Could you check a few things on this model? Use its own coordinates, in mm. Face numbers are marked on the shaded views. Round coordinates to 2 decimals unless told otherwise and drop trailing zeros. Write each loop counter-clockwise with the first axis right and the second up, starting at its lowest first coordinate (ties: lowest second). Pieces come first, ordered by that corner, then holes. Notation, with made-up numbers: M 13,43.5 L 53,43.5 A20 cw 53,73.5 Z; hole C -25,18.5 d7. An arc over 180 degrees is marked long. One line per question, with ' | ' between items. Start each with the question number.
```python
from build123d import *

# Parameters (mm, degrees)
SKETCH1_W             = 76.2
SKETCH1_H             = 50.8
SKETCH1_R             = 1.397
BOSS_EXTRUDE1_DEPTH   = 8.89
FILLET1_R             = 5.08
SKETCH2_R             = 2.370137615
CUT_EXTRUDE1_DEPTH    = 47.645493887
SKETCH3_R             = 5.08
CUT_EXTRUDE2_DEPTH    = 5.08
SKETCH4_W             = 50.8
SKETCH4_H             = 3.81
CUT_EXTRUDE3_DEPTH    = 47.645493887
FILLET2_R             = 1.905
F_6_32_TAPPED_HOLE1_D = 2.7051


with BuildPart() as part:
    # Sketch1 → Boss-Extrude1 (new body)
    with BuildSketch(Plane.XY):
        Rectangle(SKETCH1_W, SKETCH1_H)
        with Locations((-31.172764277, -20.781842852)):
            Circle(SKETCH1_R, mode=Mode.SUBTRACT)
        with Locations((31.172764277, 20.781842852)):
            Circle(SKETCH1_R, mode=Mode.SUBTRACT)
        with Locations((-31.172764277, 20.781842852)):
            Circle(SKETCH1_R, mode=Mode.SUBTRACT)
        with Locations((31.172764277, -20.781842852)):
            Circle(SKETCH1_R, mode=Mode.SUBTRACT)
    extrude(amount=BOSS_EXTRUDE1_DEPTH)

    # Fillet1
    fillet1_edges = [part.edges().sort_by_distance(p)[0] for p in [
        (38.1, -25.4, 4.445),
        (-38.1, -25.4, 4.445),
        (-38.1, 25.4, 4.445),
        (38.1, 25.4, 4.445),
    ]]
    fillet(fillet1_edges, radius=FILLET1_R)

    # Sketch2 → Cut-Extrude1 (cut, through all)
    with BuildSketch(Plane.XY.offset(8.89)):
        with Locations((19.05, 13.146852544)):
            Circle(SKETCH2_R)
        with Locations((19.05, -12.253147456)):
            Circle(SKETCH2_R)
    extrude(amount=-CUT_EXTRUDE1_DEPTH, mode=Mode.SUBTRACT)

    # Sketch3 → Cut-Extrude2 (cut)
    with BuildSketch(Plane.XY.offset(8.89)):
        with Locations((19.05, 13.146852544)):
            Circle(SKETCH3_R)
        with Locations((19.05, -12.253147456)):
            Circle(SKETCH3_R)
    extrude(amount=-CUT_EXTRUDE2_DEPTH, mode=Mode.SUBTRACT)

    # Sketch4 → Cut-Extrude3 (cut, through all)
    with BuildSketch(Plane.XY.offset(8.89)):
        with Locations((0, 23.495)):
            Rectangle(SKETCH4_W, SKETCH4_H)
    extrude(amount=-CUT_EXTRUDE3_DEPTH, mode=Mode.SUBTRACT)

    # Fillet2
    fillet2_edges = [part.edges().sort_by_distance(p)[0] for p in [
        (25.4, 21.59, 4.445),
        (-25.4, 21.59, 4.445),
    ]]
    fillet(fillet2_edges, radius=FILLET2_R)
    fillet2_2_edges = [part.edges().sort_by_distance(p)[0] for p in [
        (25.4, 25.4, 4.445),
        (-25.4, 25.4, 4.445),
    ]]
    fillet(fillet2_2_edges, radius=FILLET2_R - 0.0001)  # a hair under: the kernel refuses the full size

    # #6-32 Tapped Hole1 (through all)
    with Locations(Plane.XY.offset(8.89)):
        with Locations((-16.875568399, 1.822244587)):
            Hole(F_6_32_TAPPED_HOLE1_D / 2)


solid = part.part
```
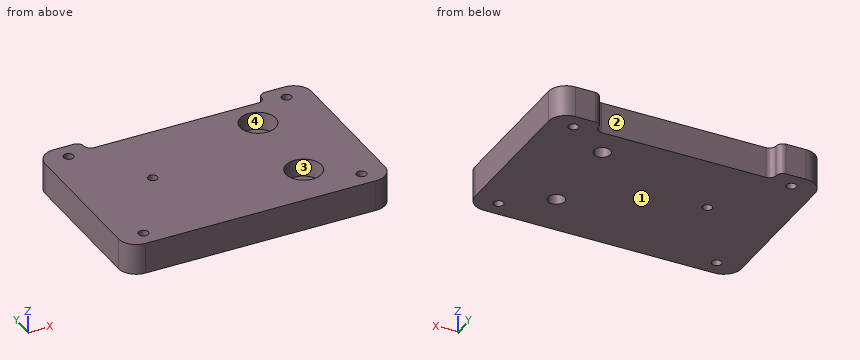
1. Suppose I cut it at B-B (z = 8). Count the separate pieces of the cut face and the enclosed holes in it, and give its area (3 significant figures).
2. Suppose I cut it at C-C (x = 9.5). Write out the boundary of the cut face in (y, z), and give its area (3 significant figures).
3. I need wall thicknesses on line 1 along Y through (x, z) = (19.05, 1.85); line 2 along Y through (x, z) = (19.05, 5.85); line 3 along X through (y, z) = (-20.5, 2). Which ranges of each line are inside material? Lowest first, please. Write a range as from..to.
4. I'm going to push flat-ended pins straight in: P1, Ø5, axis at x = 21, z = 5.5, coming from the +Y side; P2, Ø3, axis at x = 19.5, y = -11, coming from the +Z side. Where does each tip first touch, or does it pass through?
5. If we mould it in two halves opening along Y, with no side actions, what happens to the marked faces 1, 2, 3 and 4? For each: released by +Y, released by -Y, zero draft, split by the parting line, or undercut.
6. Suppose I cut it at A-A (x = 19.05). Write out the boundary of the cut face in (y, z).
Computed:
1) separate pieces: 1 | enclosed holes: 7 | area: 3,460 mm²
2) outline: M -25.4,0 L 21.59,0 L 21.59,8.89 L -25.4,8.89 Z | area: 418 mm²
3) line 1: y = -25.4..-14.62, -9.88..10.78, 15.52..21.59 | line 2: y = -25.4..-17.33, -7.17..8.07, 18.23..21.59 | line 3: x = -38.1..-32.54, -29.8..29.8, 32.54..38.1
4) P1: stops at y = 21.59 | P2: stops at z = 3.81
5) face 1: zero draft | face 2: released by +Y | face 3: undercut | face 4: undercut
6) outline: M -25.4,0 L -14.62,0 L -14.62,3.81 L -17.33,3.81 L -17.33,8.89 L -25.4,8.89 Z; M -9.88,0 L 10.78,0 L 10.78,3.81 L 8.07,3.81 L 8.07,8.89 L -7.17,8.89 L -7.17,3.81 L -9.88,3.81 Z; M 15.52,0 L 21.59,0 L 21.59,8.89 L 18.23,8.89 L 18.23,3.81 L 15.52,3.81 Z
